Verification items for the finished model (mm, model axes). Face numbers are marked on the shaded views. A direction names the side the tool comes from. Give positions to 0.01 mm unless a question says otherwise; leave off trailing zeros. Order: outer loops, then holes, each group sorted by start corner. A loop starts at its lowest first (then second) coordinate and runs counter-clockwise, first axis right, second up. Notation, with made-up numbers: (61.25, -39) - (71.25, -39) arc R34 ccw to (71.25, -8) - close; hole circle Ø5 at (6, 76). An arc over 180 degrees is marked (long way). Answer as a JSON object with one key per item and string values. Group by question number.
(1) Section check A-A (x = 0). Record the boundary of the cut face in (y, z).
(2) Section check B-B (y = 2). Record the boundary of the cut face in (x, z).
(3) Thickness scan on line 1 (Y direction, x = 0, z = 2); line 2 (X direction, y = 1, z = 6.25); line 3 (X direction, y = -1, z = 9). Record the ranges inside material, lowest first.
(4) Depth check by flat-ended pin: pin 1 Ø5.5 at (x, y) = (0, 0) entering from -Z; pin 2 Ø1.7 at (y, z) = (-4.5, 5) entering from +X; pin 3 Ø1.5 at (x, z) = (4, 4) entering from -Y; pin 4 Ø1.2 at (y, z) = (-4.5, 4) entering from -X. Enter the tip coordinate at first touch or a pass-through.
(5) Access from +Z, -Z, +X, -X, +Y, -Y to the whole of each face (thin tool, end or side, straight path). Record for the marked faces 4, 5, 6 and 7.
(6) Mould release check, pull along X, two halves, no side actions. Record for the marked faces 1, 2 and 3: +X half, -X half, draft (parallel to the pull), parting line (faces both ways), or undercut.
(7) Section check C-C (y = 4.75). Record the boundary of the cut face in (x, z).
```python
from build123d import *

# Parameters (mm, degrees)
SKETCH1_R         = 4.25
EXTRUDE1_DEPTH    = 10
SKETCH3_R         = 3.15
EXTRUDE2_DEPTH    = 11
EXTRUDE3_DEPTH    = 10
CIRPATTERN1_COUNT = 9


with BuildPart() as part:
    # Sketch1 → Extrude1 (new body)
    with BuildSketch(Plane.XY):
        Circle(SKETCH1_R)
    extrude(amount=EXTRUDE1_DEPTH)

    # Sketch3 → Extrude2 (cut, through all)
    with BuildSketch(Plane(origin=(0, 0, 0), x_dir=(-1, 0, 0), z_dir=(0, 0, -1))):
        Circle(SKETCH3_R)
    extrude(amount=-EXTRUDE2_DEPTH, mode=Mode.SUBTRACT)

    # Sketch4 → Extrude3 (add)
    with BuildSketch(Plane.XY):
        Polygon((-0.475, 5.58000953), (0.475, 5.58000953), (1.00275684, 4.13000953), (-1.00275684, 4.13000953), align=None)
    extrude3 = extrude(amount=EXTRUDE3_DEPTH)

    # CirPattern1: Extrude3 ×9 about axis
    cirpattern1_axis = Axis((0, 0, 0), (0, 0, 1))
    for i in range(1, CIRPATTERN1_COUNT):
        add(extrude3.rotate(cirpattern1_axis, i * 360 / CIRPATTERN1_COUNT))


solid = part.part
```
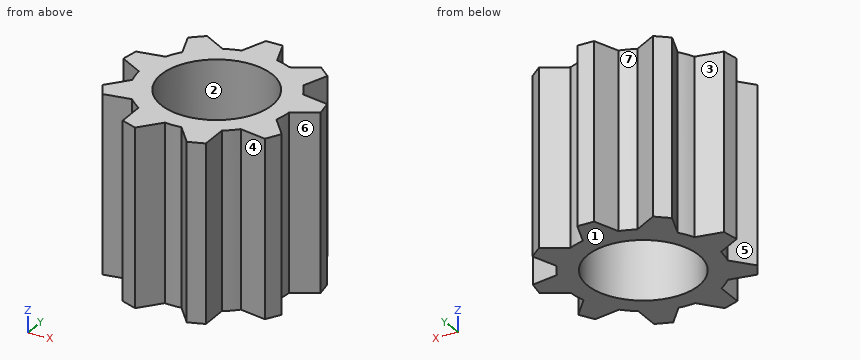
Solutions:
{
 "1": {"outline": "(-4.25, 0) - (-3.15, 0) - (-3.15, 10) - (-4.25, 10) - close; (3.15, 0) - (5.58, 0) - (5.58, 10) - (3.15, 10) - close"},
 "2": {"outline": "(-3.75, 0) - (-2.43, 0) - (-2.43, 10) - (-3.75, 10) - close; (2.43, 0) - (3.75, 0) - (3.75, 10) - (2.43, 10) - close"},
 "3": {"line 1": "y = -4.25 to -3.15, 3.15 to 5.58", "line 2": "x = -5.49 to -2.99, 2.99 to 5.49", "line 3": "x = -4.13 to -2.99, 2.99 to 4.13"},
 "4": {"pin 1": "passes through", "pin 2": "stops at x = 2.35", "pin 3": "stops at y = -3.2", "pin 4": "stops at x = -2.35"},
 "5": {"face 4": "+Z, -Z, -Y", "face 5": "+Z, -Z, -X", "face 6": "+Z, -Z, +X", "face 7": "+Z, -Z, +Y"},
 "6": {"face 1": "draft", "face 2": "undercut", "face 3": "-X half"},
 "7": {"outline": "(-0.78, 0) - (0.78, 0) - (0.78, 10) - (-0.78, 10) - close"}
}
